Autodesk Inventor part; units mm, degrees
ref_plane "YZ Plane" through (0, 0, 0) normal (1, 0, 0) x (0, 1, 0)
ref_plane "XZ Plane" through (0, 0, 0) normal (0, 1, 0) x (-1, 0, 0)
ref_plane "XY Plane" through (0, 0, 0) normal (0, 0, 1) x (1, 0, 0)
sketch "Sketch1" plane through (0, 0, 0) normal (0, 0, 1) x (1, 0, 0)
  circle A0 centre (0, 0) radius 30.15
  dimension "d0" = 60.3
extrude "Extrusion1" add sketch "Sketch1" along normal blind 200
sketch "Sketch2" plane through (0, 0, 200) normal (0, 0, 1) x (1, 0, 0)
  circle A0 centre (0, 0) radius 26.15
  dimension "d3" = 52.3
extrude "Extrusion2" cut sketch "Sketch2" against normal blind 200
sketch "Sketch3" plane through (0, 0, 0) normal (1, 0, 0) x (0, 1, 0)
  circle A0 centre (0, 50) radius 5.5
  line L0 (30.15, 0) -> (-30.15, 0)
  point P0 (0, 0)
  dimension "d6" = 11
  dimension "d7" = 50
extrude "Extrusion3" cut sketch "Sketch3" along normal through all both and the other way through all
properties part number "rura do spawania"
Part model, mm, in its own coordinate system. Give positions to 0.01 mm unless a question says otherwise; leave off trailing zeros. Write each loop counter-clockwise with the first axis right and the second up, starting at its lowest first coordinate (ties: lowest second). Pieces come first, ordered by that corner, then holes. Notation, with made-up numbers: (29, 31.25) -> (64, 31.25) arc R27 ccw to (64, 54.25) -> close; hole circle Ø3 at (43, -36). An arc over 180 degrees is marked (long way). Put each result on its own line as item: value. Start each with the question number.
Item 1: Cut at D-D (z = 92.5). List the corners of the cut face in (x, y).
Item 2: Cut at C-C (y = 16.5). List the corners of the cut face in (x, z), then the cut area to 3 significant figures.
Item 3: Pin check, flat tips, straight feed: pin 1 Ø14.5 at (y, z) = (0, 50) entering from -X; pin 2 Ø8 at (x, z) = (5.5, 60.5) entering from +Y; pin 3 Ø6 at (x, z) = (-6, 31) entering from -Y; pin 4 Ø1 at (y, z) = (17.5, 118) entering from +X. Stop position of each tip, or through.
Item 4: Wall check: L1, parallel to Y at x = 0, z = 144; L2, parallel to X at y = 21, z = 82. Give the ranges that are in metal, low to high. Write a range as [from, to].
Item 5: Cut at B-B (x = 0). List the corners of the cut face in (y, z).
Item 6: Cut at A-A (y = 0). List the corners of the cut face in (x, z), then the cut area to 3 significant figures.
Item 7: Pull direction Z, two halves, no side cores. Call faces 1 (the face through (-9, 25, 0)), 2 (the face through (-9, 25, 200)), 3 (the face through (27.825, -0.716, 44.547)): pulls with the +Z half, pulls with the -Z half, needs draft (parallel to the pull), parting line crosses it, or undercut.
Answer list:
1. outline: circle Ø60.3 at (0, 0); hole circle Ø52.3 at (0, 0)
2. outline: (-25.23, 0) -> (-20.29, 0) -> (-20.29, 200) -> (-25.23, 200) -> close; (20.29, 0) -> (25.23, 0) -> (25.23, 200) -> (20.29, 200) -> close
2. area: 1,980 mm2
3. pin 1: stops at x = -30.15
3. pin 2: stops at y = 30.11
3. pin 3: stops at y = -30
3. pin 4: stops at x = 24.9
4. L1: y = [-30.15, -26.15], [26.15, 30.15]
4. L2: x = [-21.63, -15.58], [15.58, 21.63]
5. outline: (-30.15, 0) -> (-26.15, 0) -> (-26.15, 200) -> (-30.15, 200) -> close; (26.15, 0) -> (30.15, 0) -> (30.15, 200) -> (26.15, 200) -> close
6. outline: (-30.15, 0) -> (-26.15, 0) -> (-26.15, 44.5) -> (-30.15, 44.5) -> close; (-30.15, 55.5) -> (-26.15, 55.5) -> (-26.15, 200) -> (-30.15, 200) -> close; (26.15, 0) -> (30.15, 0) -> (30.15, 44.5) -> (26.15, 44.5) -> close; (26.15, 55.5) -> (30.15, 55.5) -> (30.15, 200) -> (26.15, 200) -> close
6. area: 1,510 mm2
7. face 1: pulls with the -Z half
7. face 2: pulls with the +Z half
7. face 3: undercut
